Could you check a few things on this model? Use its own coordinates, in mm. A direction names the side the tool comes from. Round coordinates to 2 decimals unless told otherwise and drop trailing zeros. Order: outer loops, then holes, each group sorted by start corner. A loop starts at its lowest first (then second) coordinate and runs counter-clockwise, first axis right, second up. Notation, with made-up numbers: (57.25, 83) - (111.25, 83) arc R11 ccw to (111.25, 95) - close; hole circle Ø7 at (87.25, 24). An arc over 180 degrees is marked (long way). Use one line per item in the form item = value.
from build123d import *

# Parameters (mm, degrees)
SKETCH_1_W          = 92
SKETCH_1_H          = 49
EXTRUDE_1_DEPTH     = 22
SKETCH_2_W          = 6
SKETCH_2_H          = 10
EXTRUDE_2_DEPTH     = 4
CUT_EXTRUDE_2_DEPTH = 91
SKETCH_5_R          = 1.5
EXTRUDE_3_DEPTH     = 5


with BuildPart() as part:
    # 草图1 → 凸台-拉伸1 (new body)
    with BuildSketch(Plane(origin=(0, 0, 0), x_dir=(1, 0, 0), z_dir=(0, 1, 0))):
        with Locations((-1.545219638, 10.208010336)):
            Rectangle(SKETCH_1_W, SKETCH_1_H)
    extrude(amount=EXTRUDE_1_DEPTH)

    # 草图2 → 凸台-拉伸2 (add)
    with BuildSketch(Plane(origin=(0, 0, -34.708010336), x_dir=(-1, 0, 0), z_dir=(0, 0, -1))):
        with Locations((-39.454780362, 11)):
            Rectangle(SKETCH_2_W, SKETCH_2_H)
    extrude(amount=EXTRUDE_2_DEPTH)

    # 草图3 → 切除-拉伸2 (cut, through all)
    with BuildSketch(Plane(origin=(42.454780362, 0, 0), x_dir=(0, 0, -1), z_dir=(1, 0, 0))):
        Polygon((38.708010336, 16), (34.708010336, 16), (38.708010336, 13.690598923), align=None)
        Polygon((38.708010336, 13.690598923), (34.708010336, 6), (38.708010336, 6), align=None)
    extrude(amount=-CUT_EXTRUDE_2_DEPTH, mode=Mode.SUBTRACT)

    # 草图4 → 旋转1 (revolve)
    with BuildSketch(Plane(origin=(0, 0, -34.708010336), x_dir=(-1, 0, 0), z_dir=(0, 0, -1))):
        with BuildLine():
            Line((-34.454780362, 11), (-34.454780362, 12))
            ThreePointArc((-34.454780362, 12), (-33.454780362, 11), (-34.454780362, 10))
            Line((-34.454780362, 10), (-34.454780362, 11))
        make_face()
    revolve(axis=Axis((34.454780362, 11, -34.708010336), (0, 1, 0)))

    # 草图5 → 凸台-拉伸3 (add)
    with BuildSketch(Plane.XY.offset(14.291989664)):
        with Locations((42.72658272, 13)):
            Circle(SKETCH_5_R)
        with Locations((42.72658272, 9)):
            Circle(SKETCH_5_R)
    extrude(amount=EXTRUDE_3_DEPTH)


solid = part.part
Item 1: I need wall thicknesses on L1, parallel to Z at x = 8.5, y = 4.25. Which ranges of the line are inside material? Lowest first, please.
Found:
L1 = -34.71 to 14.29
Item 2: Imagine slicing it at C-C on y = 19. Please give me the cut outline in (x, z).
Found:
outline = (-47.55, -34.71) - (44.45, -34.71) - (44.45, 14.29) - (-47.55, 14.29) - close
Item 3: Imagine slicing it at A-A on x = 38.5. Please give me the cut outline in (y, z).
Found:
outline = (0, -34.71) - (6, -34.71) - (13.69, -38.71) - (16, -34.71) - (22, -34.71) - (22, 14.29) - (0, 14.29) - close
Item 4: Will these pins go through, and if not, where does the flat tip stop? P1, Ø6.5, axis at x = -19, y = 16.5, coming from the +Z side; P2, Ø2, axis at x = 9.5, y = 8, coming from the -Z side; P3, Ø4.5, axis at y = 11, z = -37, coming from the +X side.
Found:
P1 = 14.29
P2 = -34.71
P3 = 42.45
Item 5: Imagine slicing it at B-B on y = 9. Please give me the cut outline in (x, z), plus the area to 3 significant figures.
Found:
outline = (-47.55, -34.71) - (36.45, -34.71) - (36.45, -36.27) - (42.45, -36.27) - (42.45, -34.71) - (44.45, -34.71) - (44.45, 14.29) - (44.23, 14.29) - (44.23, 19.29) - (41.23, 19.29) - (41.23, 14.29) - (-47.55, 14.29) - close
area = 4,530 mm2
Item 6: For faces 4 (the face through (41.23, 13.07, 16.76)), 5 (the face through (42.455, 12, -36)), 6 (the face through (-2, 22, -11)), which set-ups out of +Z, -Z, +X, -X, +Y, -Y let a thin tool reach every point of the face, with its end or its side?
Found:
face_4 = +Z
face_5 = -Z, +X, +Y, -Y
face_6 = +Z, -Z, +X, -X, +Y
Item 7: Imagine slicing it at D-D on x = 22. Please give me the cut outline in (y, z), plus the area to 3 significant figures.
Found:
outline = (0, -34.71) - (22, -34.71) - (22, 14.29) - (0, 14.29) - close
area = 1,080 mm2
Item 8: If we mould it in two halves opening along Y, with no side actions, what happens to faces 1 (the face through (-2, 0, -11)), 2 (the face through (41.536, 8.087, 16.757)), 3 (the face through (-2, 11, -34.708))? For each: released by +Y, released by -Y, zero draft, split by the parting line, or undercut.
Found:
face_1 = released by -Y
face_2 = undercut
face_3 = zero draft
